Could you check a few things on this model? Use its own coordinates, in mm. Face numbers are marked on the shaded views. Coordinates: 2 decimals unless noted, no trailing zeros. Write each loop counter-clockwise with the first axis right and the second up, starting at its lowest first coordinate (ties: lowest second). Pieces come first, ordered by that corner, then holes. Notation, with made-up numbers: (-22, 22.5) - (11, 22.5) arc R23 cw to (11, 39.5) - close; hole circle Ø9 at (16, 88). An arc over 180 degrees is marked (long way). Write item = value, one per line. Start each with the question number.
```python
from build123d import *

# Parameters (mm, degrees)
BOSS_EXTRUDE1_DEPTH = 10
SKETCH2_W           = 20
SKETCH2_H           = 20
BOSS_EXTRUDE2_DEPTH = 26.2
BOSS_EXTRUDE3_DEPTH = 20


with BuildPart() as part:
    # Sketch1 → Boss-Extrude1 (new, symmetric)
    with BuildSketch(Plane.XY):
        with BuildLine():
            Line((45.962666587, 38.567256581), (30.641777725, 25.711504387))
            ThreePointArc((30.641777725, 25.711504387), (0, 40), (-30.641777725, 25.711504387))
            Line((-30.641777725, 25.711504387), (-45.962666587, 38.567256581))
            ThreePointArc((-45.962666587, 38.567256581), (0, 60), (45.962666587, 38.567256581))
        make_face()
    extrude(amount=BOSS_EXTRUDE1_DEPTH, both=True)

    # Sketch2 → Boss-Extrude2 (add)
    with BuildSketch(Plane(origin=(0, 0, 0), x_dir=(0, 0, 1), z_dir=(-0.6427876096865383, -0.7660444431189791, 0))):
        with Locations((0, 50)):
            Rectangle(SKETCH2_W, SKETCH2_H)
    boss_extrude2 = extrude(amount=BOSS_EXTRUDE2_DEPTH)

    # Mirror1: Boss-Extrude2 across plane
    add(boss_extrude2.mirror(Plane.ZY))

    # Sketch3 → Boss-Extrude3 (add)
    with BuildSketch(Plane(origin=(0, 0, -10), x_dir=(-1, 0, 0), z_dir=(0, 0, -1))):
        Polygon((47.482813099, 5.641139978), (62.803701961, 18.496892171), (68.765030296, 11.392457711), (53.444141434, -1.463294483), align=None)
        Polygon((-53.444141434, -1.463294483), (-68.765030296, 11.392457711), (-62.803701961, 18.496892171), (-47.482813099, 5.641139978), align=None)
    extrude(amount=-BOSS_EXTRUDE3_DEPTH)


solid = part.part
```
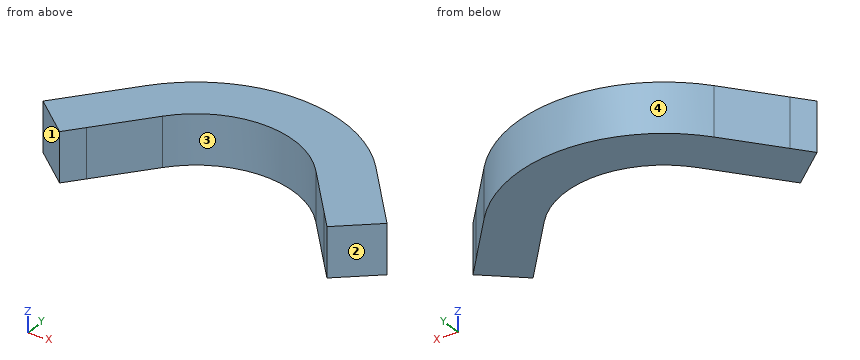
1) Thinking about a two-plate mould opening in X: for the marked faces 1, 2, 3 and 4, which applies, +X half, -X half, draft (parallel to the pull), parting line (faces both ways), or undercut?
2) For P1, Ø2, axis at x = 38, z = -5, coming from the +Y side; P2, Ø1.5, axis at x = -39, z = 0.5, coming from the +Y side; P3, Ø2, axis at x = -6, z = -6, coming from the +Y side, each with a flat end and sliding along its axis, tell me the tip position at first contact or that it passes through.
3) Suppose I cut it at B-B on y = 29.5. Please give me the cut outline in (x, z).
4) Suppose I cut it at A-A on z = -2.5. Please give me the cut outline in (x, y).
5) If I drill on probe 1 along Y at (x, z) = (-0.5, -3.5); probe 2 along X at (y, z) = (21.5, -9); probe 3 along X at (y, z) = (30, -3), over which ranges is the centre line in solid material (lowest first)? Write a range as [from, to].
6) Suppose I cut it at D-D on y = 49.5. Please give me the cut outline in (x, z).
7) Suppose I cut it at C-C on x = 34. Please give me the cut outline in (y, z).
Reply:
q1.face_1 = -X half
q1.face_2 = +X half
q1.face_3 = undercut
q1.face_4 = parting line
q2.P1 = 47.23
q2.P2 = 46.23
q2.P3 = 59.79
q3.outline = (-53.57, -10) - (-27.01, -10) - (-27.01, 10) - (-53.57, 10) - close; (27.01, -10) - (53.57, -10) - (53.57, 10) - (27.01, 10) - close
q4.outline = (-68.77, 11.39) - (-53.44, -1.46) - (-30.64, 25.71) arc R40 cw to (30.64, 25.71) - (53.44, -1.46) - (68.77, 11.39) - (45.96, 38.57) arc R60 ccw to (-45.96, 38.57) - close
q5.probe_1 = [40, 60]
q5.probe_2 = [-60.28, -34.18], [34.18, 60.28]
q5.probe_3 = [-53.15, -26.46], [26.46, 53.15]
q6.outline = (-33.91, -10) - (33.91, -10) - (33.91, 10) - (-33.91, 10) - close
q7.outline = (21.71, -10) - (49.44, -10) - (49.44, 10) - (21.71, 10) - close
